from build123d import *

# Parameters (mm, degrees)
BOSS_EXTRU_1_DEPTH      = 530
ESQUISSE2_W             = 68
ESQUISSE2_H             = 61
ENL_V_MAT_EXTRU_1_DEPTH = 9
ESQUISSE3_R             = 2.5
ENL_V_MAT_EXTRU_2_DEPTH = 7


with BuildPart() as part:
    # Esquisse1 → Boss.-Extru.1 (new body)
    with BuildSketch(Plane.XY):
        Polygon((0, 0), (83, 0), (83, 7), (46, 7), (46, 68), (37, 68), (37, 7), (0, 7), align=None)
    extrude(amount=BOSS_EXTRU_1_DEPTH)

    # Esquisse2 → Enlèv. mat.-Extru.1 (cut)
    with BuildSketch(Plane.ZY.offset(-37)):
        with Locations((34, 37.5)):
            Rectangle(ESQUISSE2_W, ESQUISSE2_H)
        with Locations((496, 37.5)):
            Rectangle(ESQUISSE2_W, ESQUISSE2_H)
    extrude(amount=-ENL_V_MAT_EXTRU_1_DEPTH, mode=Mode.SUBTRACT)

    # Esquisse3 → Enlèv. mat.-Extru.2 (cut)
    with BuildSketch(Plane.XZ):
        with Locations(Location((29.5, 80, 0), (0, 0, 270))):
            Circle(ESQUISSE3_R)
        with Locations(Location((53.5, 80, 0), (0, 0, 90))):
            Circle(ESQUISSE3_R)
        with Locations(Location((29.5, 180, 0), (0, 0, 270))):
            Circle(ESQUISSE3_R)
        with Locations(Location((53.5, 180, 0), (0, 0, 90))):
            Circle(ESQUISSE3_R)
        with Locations(Location((29.5, 280, 0), (0, 0, 270))):
            Circle(ESQUISSE3_R)
        with Locations(Location((53.5, 280, 0), (0, 0, 90))):
            Circle(ESQUISSE3_R)
        with Locations(Location((29.5, 380, 0), (0, 0, 270))):
            Circle(ESQUISSE3_R)
        with Locations(Location((53.5, 380, 0), (0, 0, 90))):
            Circle(ESQUISSE3_R)
        with Locations(Location((29.5, 480, 0), (0, 0, 270))):
            Circle(ESQUISSE3_R)
        with Locations(Location((53.5, 480, 0), (0, 0, 90))):
            Circle(ESQUISSE3_R)
    extrude(amount=-ENL_V_MAT_EXTRU_2_DEPTH, mode=Mode.SUBTRACT)


solid = part.part
Can you work these out from the model? Positions are in its coordinate system, mm. A direction names the side the tool comes from. Round coordinates to 2 decimals unless told otherwise and drop trailing zeros. Write each loop counter-clockwise with the first axis right and the second up, starting at its lowest first coordinate (ties: lowest second). Pieces come first, ordered by that corner, then holes. Notation, with made-up numbers: (-27, 45) -> (29, 45) arc R23 cw to (29, 55) -> close; hole circle Ø7 at (30, 63). An arc over 180 degrees is marked (long way). One line per question, with ' | ' between items. Start each with the question number.
1) I need wall thicknesses on line 1 (Z direction, x = 53, y = 4); line 2 (X direction, y = 3, z = 180); line 3 (Y direction, x = 18.5, z = 309). Which ranges of each line are inside material? Lowest first, please. Write a range as [from, to].
2) I'm going to push flat-ended pins straight in: P1, Ø18.5, axis at y = 30, z = 221, coming from the -X side; P2, Ø10, axis at x = 22, z = 370.5, coming from the +Y side; P3, Ø4, axis at x = 29.5, z = 80, coming from the -Y side; P4, Ø10, axis at x = 42.5, y = 32, coming from the -Z side. Where does each tip first touch, or does it pass through?
3) On a 3-axis mill with a long thin cutter (end or side, diameter ignored), from which of +Z, -Z, +X, -X, +Y, -Y can I reach the whole of each face in a straight line? I mean faces 1 (the flat face through (37, 38, 262)), 2 (the flat face through (41, 37, 462)), 3 (the flat face through (46, 37, 262)). Say none if no direction works.
4) Suppose I cut it at B-B on x = 76. Write out the boundary of the cut face in (y, z).
5) Suppose I cut it at A-A on z = 119. Write out the boundary of the cut face in (x, y), then the cut area to 3 significant figures.
6) Suppose I cut it at C-C on y = 55.5. Write out the boundary of the cut face in (x, z), then the cut area to 3 significant figures.
Return value:
1) line 1: z = [0, 77.55], [82.45, 177.55], [182.45, 277.55], [282.45, 377.55], [382.45, 477.55], [482.45, 530] | line 2: x = [0, 27], [32, 51], [56, 83] | line 3: y = [0, 7]
2) P1: stops at x = 37 | P2: stops at y = 7 | P3: passes through | P4: stops at z = 68
3) face 1: +Z, -Z, -X, +Y | face 2: +Z, +X, -X, +Y | face 3: +Z, -Z, +X, +Y
4) outline: (0, 0) -> (7, 0) -> (7, 530) -> (0, 530) -> close
5) outline: (0, 0) -> (83, 0) -> (83, 7) -> (46, 7) -> (46, 68) -> (37, 68) -> (37, 7) -> (0, 7) -> close | area: 1,130 mm2
6) outline: (37, 68) -> (46, 68) -> (46, 462) -> (37, 462) -> close | area: 3,550 mm2
